from build123d import *

# Parameters (mm, degrees)
CHAMFER1_SIZE = 0.1


with BuildPart() as part:
    # Sketch1 → Revolve1 (revolve)
    with BuildSketch(Plane(origin=(0, 0, 0), x_dir=(0, 0, -1), z_dir=(1, 0, 0)), mode=Mode.PRIVATE) as revolve1_sk:
        Polygon((-1.2, 5), (2, 5), (2, 4.510995713), (1.660325371, 4.510995713), (1.660325371, 3.031838511), (2, 3.031838511), (2, 2.5), (-2, 2.5), (-2, 3.031838511), (-1.660325371, 3.031838511), (-1.660325371, 4.510995713), (-2, 4.510995713), (-2, 5.8), (-1.2, 5.8), align=None)
    revolve(revolve1_sk.sketch.rotate(Axis((0, 0, -19.078271996), (0, 0, 1)), 90), axis=Axis((0, 0, -19.078271996), (0, 0, 1)))

    # Chamfer1
    chamfer1_edges = [part.edges().sort_by_distance(p)[0] for p in [
        (3.031838511, 0, 2),
        (4.510995713, 0, 2),
        (5.8, 0, 2),
        (5.8, 0, 1.2),
        (5, 0, -2),
        (4.510995713, 0, -2),
        (3.031838511, 0, -2),
        (2.5, 0, -2),
        (2.5, 0, 2),
    ]]
    chamfer(chamfer1_edges, length=CHAMFER1_SIZE)


solid = part.part
The listing builds one solid part. Answer for the finished solid, in the listing's coordinates (mm). Round coordinates to 2 decimals unless told otherwise and drop trailing zeros. Order: outer loops, then holes, each group sorted by start corner. A loop starts at its lowest first (then second) coordinate and runs counter-clockwise, first axis right, second up. Notation, with made-up numbers: M 4,48 L 54,48 A8 cw 54,60 Z; hole C -19,65.25 d7. An arc over 180 degrees is marked long. Answer in a Markdown table with one row per item. Add a question column.
1) The part is cut by section A-A on z = -0.8. Determine the outline of the cut face in (x, y), plus the area to 3 significant figures.
2) Consider line 1 along Y through (x, z) = (0, -1.8); line 2 along Y through (x, z) = (0, -0.15); line 3 along Y through (x, z) = (1, 1.8). Determine where each line is inside the solid, lowest interval first. Write a range as from..to.
3) Determine the mould class of faces 1 (the face through (5.794, -0.255, 1.596)), 2 (the face through (2.5, -0.1, 0)), 3 (the face through (5, 0, 2)) for opening direction X: pulls with the +X half, pulls with the -X half, needs draft (parallel to the pull), parting line crosses it, or undercut.
Findings below:
| question | item | result |
|---|---|---|
| 1 | outline | C 0,0 d10; hole C 0,0 d5 |
| 1 | area | 58.9 mm² |
| 2 | line 1 | y = -5..-4.51, -3.03..-2.5, 2.5..3.03, 4.51..5 |
| 2 | line 2 | y = -5..-2.5, 2.5..5 |
| 2 | line 3 | y = -5.71..-4.4, -2.86..-2.29, 2.29..2.86, 4.4..5.71 |
| 3 | face 1 | parting line crosses it |
| 3 | face 2 | undercut |
| 3 | face 3 | needs draft |
